from build123d import *

# Parameters (mm, degrees)
BOSS_EXTRUDE1_DEPTH = 22.5
BOSS_EXTRUDE2_START = 6.5
SKETCH2_R           = 5
BOSS_EXTRUDE2_DEPTH = 10
BOSS_EXTRUDE3_START = -16.5
SKETCH2_2_R         = 5
BOSS_EXTRUDE3_DEPTH = 10
SKETCH3_R           = 4
BOSS_EXTRUDE4_DEPTH = 6
SKETCH4_R           = 4
CUT_EXTRUDE1_DEPTH  = 100.824444172


with BuildPart() as part:
    # Sketch1 → Boss-Extrude1 (new, symmetric)
    with BuildSketch(Plane(origin=(0, 0, 0), x_dir=(0, 0, -1), z_dir=(1, 0, 0))):
        Polygon((-16, 0.019237886), (16, 0.019237886), (16.011106999, 60.019237886), (6.011106999, 60.019237886), (-9, 34.019237886), (-9, 12.019237886), (-16, 12.019237886), align=None)
    extrude(amount=BOSS_EXTRUDE1_DEPTH, both=True)

    # Sketch2 → Boss-Extrude2 (add)
    with BuildSketch(Plane(origin=(0, 0, 0), x_dir=(0, 0, -1), z_dir=(1, 0, 0)).offset(BOSS_EXTRUDE2_START)):
        with BuildLine():
            Line((16.006293966, 34.019238332), (16.011106999, 60.019237886))
            Line((16.011106999, 60.019237886), (46.011106999, 60.019237886))
            ThreePointArc((46.011106999, 60.019237886), (55.965350951, 50.974762528), (47.913412075, 40.201843354))
            Line((47.913412075, 40.201843354), (16.006293966, 34.019238332))
        make_face()
        with Locations((46.011106999, 50.019237886)):
            Circle(SKETCH2_R, mode=Mode.SUBTRACT)
    extrude(amount=BOSS_EXTRUDE2_DEPTH)

    # Sketch2<2> → Boss-Extrude3 (add)
    with BuildSketch(Plane(origin=(0, 0, 0), x_dir=(0, 0, -1), z_dir=(1, 0, 0)).offset(BOSS_EXTRUDE3_START)):
        with BuildLine():
            Line((16.006293966, 34.019238332), (16.011106999, 60.019237886))
            Line((16.011106999, 60.019237886), (46.011106999, 60.019237886))
            ThreePointArc((46.011106999, 60.019237886), (55.965350951, 50.974762528), (47.913412075, 40.201843354))
            Line((47.913412075, 40.201843354), (16.006293966, 34.019238332))
        make_face()
        with Locations((46.011106999, 50.019237886)):
            Circle(SKETCH2_2_R, mode=Mode.SUBTRACT)
    extrude(amount=BOSS_EXTRUDE3_DEPTH)

    # Sketch3 → Boss-Extrude4 (add, symmetric)
    with BuildSketch(Plane(origin=(0, 0, 0), x_dir=(0, 0, -1), z_dir=(1, 0, 0))):
        with BuildLine():
            Line((6.011106999, 60.019237886), (-9, 34.019237886))
            Line((-9, 34.019237886), (-33.705019764, 54.660061974))
            ThreePointArc((-33.705019764, 54.660061974), (-35.89708202, 67.430869171), (-23.643692341, 71.644311323))
            Line((-23.643692341, 71.644311323), (6.011106999, 60.019237886))
        make_face()
        with Locations((-27.293408528, 62.334124872)):
            Circle(SKETCH3_R, mode=Mode.SUBTRACT)
    extrude(amount=BOSS_EXTRUDE4_DEPTH, both=True)

    # Sketch4 → Cut-Extrude1 (cut, through all)
    with BuildSketch(Plane.XY.offset(9)):
        with Locations((-13.5, 24.019237886)):
            Circle(SKETCH4_R)
        with Locations((13.5, 24.019237886)):
            Circle(SKETCH4_R)
    extrude(amount=-CUT_EXTRUDE1_DEPTH, mode=Mode.SUBTRACT)


solid = part.part
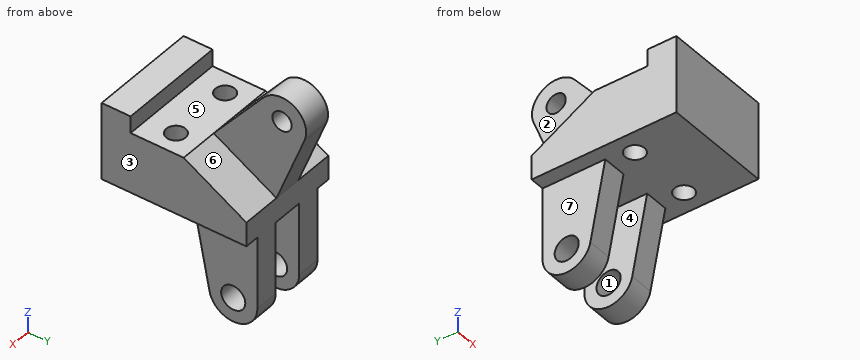
Input: part model. Units: mm. Frame: model coordinates. Face numbers are marked on the shaded views. A direction names the side the tool comes from. Coordinates: 2 decimals unless noted, no trailing zeros. Loops run counter-clockwise (first coordinate to the right, second up) from the corner with the lowest first, then second, coordinate; pieces in that order, holes last.
Q1. Cut plane A-A (z = -17.5). Output: boundary loops of the cut face in (x, y), then the cut area to 3 significant figures.
Q2. Cut plane C-C (x = 8). Output: boundary loops of the cut face in (y, z).
Q3. Material intervals for line 1 (Y direction, x = 18, z = -6); line 2 (Y direction, x = 15.5, z = 2); line 3 (X direction, y = 42.5, z = -41.5), sorted ascending.
Q4. Contact query for flat-ended pins moving along their axis: pin 1 (6 mm diameter, centred on x = -10.5, y = 32, fed in from +Z); pin 2 (13 mm diameter, centred on x = -8, y = 7.5, fed in from +Z); pin 3 (3 mm diameter, centred on y = 17, z = -18, fed in from +X); pin 4 (12 mm diameter, centred on y = 50, z = 27.5, fed in from -X). Output: stop coordinate, or through.
Q5. Cut plane B-B (x = 13.5). Output: boundary loops of the cut face in (y, z), then the cut area to 3 significant figures.
Q6. Set-up query: the marked faces 5, 6 and 7. Return all of +Z, -Z, +X, -X, +Y, -Y with unobstructed straight access to the full face (end or side cutting, diameter ignored); none if empty.
Q7. Draft query along X for the marked faces 1, 2, 3 and 4. Return one class per face: +X half, -X half, draft (parallel to the pull), parting line (faces both ways), or undercut.
Q8. Cut plane D-D (z = 7.5). Output: boundary loops of the cut face in (x, y), then the cut area to 3 significant figures.
Working result:
1. outline: (-16.5, 34.31) - (-6.5, 34.31) - (-6.5, 60.02) - (-16.5, 60.02) - close; (6.5, 34.31) - (16.5, 34.31) - (16.5, 60.02) - (6.5, 60.02) - close
1. area: 514 mm2
2. outline: (0.02, -16) - (34.02, -16.01) - (40.2, -47.91) arc R10 ccw to (60.02, -46.01) - (60.02, -6.01) - (34.02, 9) - (12.02, 9) - (12.02, 16) - (0.02, 16) - close; hole circle Ø10 at (50.02, -46.01)
3. line 1: y = 0.02 to 60
3. line 2: y = 0.02 to 20.56, 27.48 to 46.14
3. line 3: x = -16.5 to -6.5, 6.5 to 16.5
4. pin 1: stops at z = 9
4. pin 2: stops at z = 16
4. pin 3: passes through
4. pin 4: stops at x = -6
5. outline: (0.02, -16) - (20.02, -16) - (20.02, 9) - (12.02, 9) - (12.02, 16) - (0.02, 16) - close; (28.02, -16.01) - (34.02, -16.01) - (40.2, -47.91) arc R10 ccw to (60.02, -46.01) - (60.02, -6.01) - (34.02, 9) - (28.02, 9) - close; hole circle Ø10 at (50.02, -46.01)
5. area: 1,960 mm2
6. face 5: +Z, +X, -X
6. face 6: +Z, +X, +Y
6. face 7: -Z, -X, +Y, -Y
7. face 1: draft
7. face 2: -X half
7. face 3: +X half
7. face 4: undercut
8. outline: (-22.5, 0.02) - (22.5, 0.02) - (22.5, 36.62) - (6, 36.62) - (6, 65.32) - (-6, 65.32) - (-6, 36.62) - (-22.5, 36.62) - close; hole circle Ø8 at (-13.5, 24.02); hole circle Ø8 at (13.5, 24.02)
8. area: 1,890 mm2
